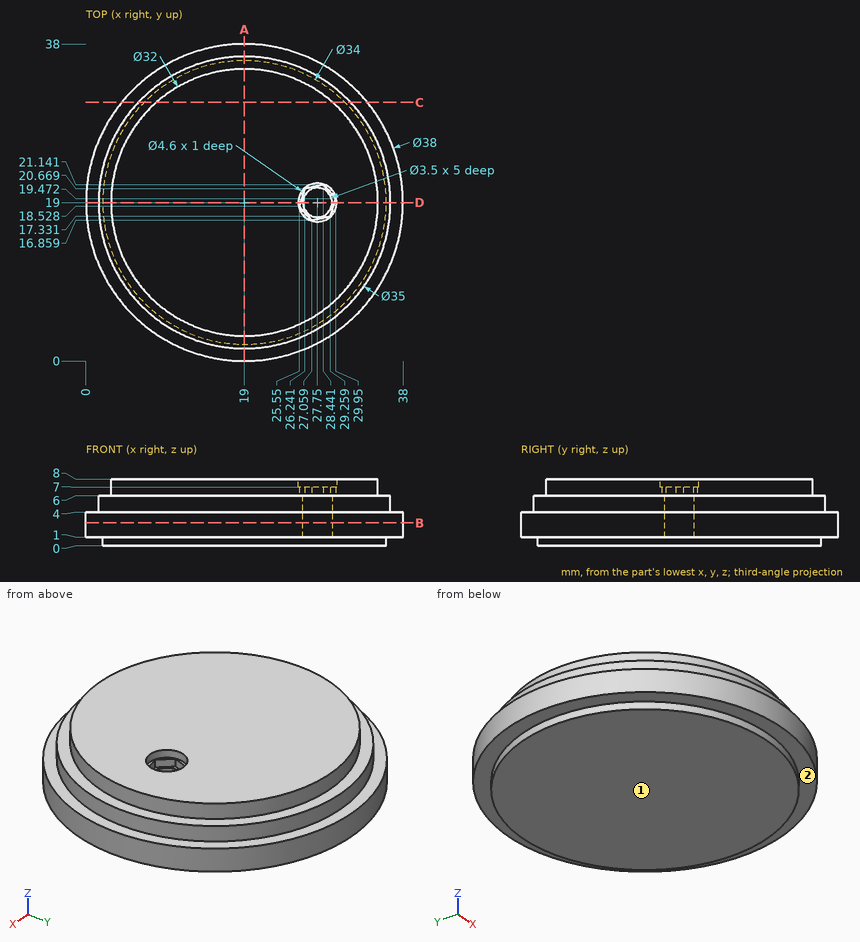
Input: dimensioned drawing with shaded views. Units: mm. Origin: part minimum x, y, z. A direction names the side the tool comes from. Give positions to 0.01 mm unless a question says otherwise; leave off trailing zeros. Order: outer loops, then holes, each group sorted by start corner. A loop starts at its lowest first (then second) coordinate and runs counter-clockwise, first axis right, second up.
(1) Section query C-C (y = 31). Return the cut outline in (x, z), plus the area to 3 significant figures.
(2) Material intervals for line 1 along Y through (x, z) = (19.5, 6.75); line 2 along Y through (x, z) = (27.75, 7.7) (1 decimal); line 3 along X through (y, z) = (14, 7.5), sorted ascending.
(3) Access query for the marked faces 1 and 2. Directions: +Z, -Z, +X, -X, +Y, -Y. A direction counts if a zero-diameter tool reaches every point of the face in a straight line with its end or side. Return the directions, or none.
(4) Section query A-A (x = 19). Return the cut outline in (y, z).
(5) Contact query for flat-ended pins moving along their axis: P1, Ø1.5, axis at x = 28.5, z = 6.5, coming from the -Y side (1 decimal); P2, Ø2, axis at x = 19.5, z = 6.5, coming from the +Y side; P3, Ø1.5, axis at y = 5.5, z = 5.5, coming from the +X side (1 decimal). Output: stop coordinate, or through.
(6) Section query D-D (y = 19). Return the cut outline in (x, z), plus the area to 3 significant figures.
(7) Section query B-B (z = 2.75). Return the cut outline in (x, y).
Outcome:
1. outline: (4.27, 1) - (6.96, 1) - (6.96, 0) - (31.04, 0) - (31.04, 1) - (33.73, 1) - (33.73, 4) - (31.74, 4) - (31.74, 6) - (29.58, 6) - (29.58, 8) - (8.42, 8) - (8.42, 6) - (6.26, 6) - (6.26, 4) - (4.27, 4) - close
1. area: 206 mm2
2. line 1: y = 3.01 to 34.99
2. line 2: y = 5.6 to 16.7, 21.3 to 32.4
2. line 3: x = 3.8 to 34.2
3. face 1: -Z, +X, -X, +Y, -Y
3. face 2: -Z
4. outline: (0, 1) - (2, 1) - (2, 0) - (36, 0) - (36, 1) - (38, 1) - (38, 4) - (36.5, 4) - (36.5, 6) - (35, 6) - (35, 8) - (3, 8) - (3, 6) - (1.5, 6) - (1.5, 4) - (0, 4) - close
5. P1: stops at y = 4
5. P2: stops at y = 36.5
5. P3: stops at x = 31
6. outline: (0, 1) - (2, 1) - (2, 0) - (36, 0) - (36, 1) - (38, 1) - (38, 4) - (36.5, 4) - (36.5, 6) - (35, 6) - (35, 8) - (30.05, 8) - (30.05, 7) - (29.8, 7) - (29.8, 6) - (29.5, 6) - (29.5, 1) - (26, 1) - (26, 6) - (25.7, 6) - (25.7, 7) - (25.45, 7) - (25.45, 8) - (3, 8) - (3, 6) - (1.5, 6) - (1.5, 4) - (0, 4) - close
6. area: 256 mm2
7. outline: circle Ø38 at (19, 19); hole circle Ø3.5 at (27.75, 19)
